Part model, mm, in its own coordinate system. Face numbers are marked on the shaded views. A direction names the side the tool comes from. Give positions to 0.01 mm unless a question says otherwise; leave off trailing zeros. Order: outer loops, then holes, each group sorted by start corner. A loop starts at its lowest first (then second) coordinate and runs counter-clockwise, first axis right, second up. Notation, with made-up numbers: (88, 82) -> (122, 82) arc R28 cw to (122, 107) -> close; hole circle Ø11 at (-32, 84). An arc over 180 degrees is marked (long way). Write item = value, one per line. Start each with the question number.
Item 1: Band-saw the part on D-D on y = -10. Write the cut outline in (x, z).
Item 2: Tool access for the marked faces 1 and 2: list every direction of +Z, -Z, +X, -X, +Y, -Y with a clear straight run to the whole face (end or side of a thin tool).
Item 3: Band-saw the part on C-C on z = 2. Count the separate pieces of the cut face and the enclosed holes in it, plus the area to 3 significant figures.
Item 4: Drill centre lines: line 1 along Y through (x, z) = (18.5, 1.5); line 2 along Y through (x, z) = (19.5, 1); line 3 along X through (y, z) = (6, 2.5). Where is each one in solid material? Low to high.
Item 5: Band-saw the part on A-A on y = 0. Write the cut outline in (x, z), plus the area to 3 significant figures.
Item 6: Flat gauge pins, fed straight in: P1, Ø5.5, axis at x = -19.05, y = 0, coming from the +Z side; P2, Ø3, axis at x = -21.5, z = 4, coming from the +Y side; P3, Ø2, axis at x = 13, y = 21.5, coming from the -Z side; P4, Ø7, axis at x = -3.5, y = -3, coming from the +Z side. Where does each tip first touch, or does it go through?
```python
from build123d import *

# Parameters (mm, degrees)
SKETCH1_R           = 30.5
SKETCH1_R_2         = 1.78
BOSS_EXTRUDE1_DEPTH = 3.1
SKETCH2_R           = 12.35
BOSS_EXTRUDE2_DEPTH = 4.1
SKETCH3_R           = 11.25
CUT_EXTRUDE1_DEPTH  = 1.5
SKETCH4_R           = 1.25
SKETCH4_R_2         = 3.1
CUT_EXTRUDE2_DEPTH  = 6.7


with BuildPart() as part:
    # Sketch1 → Boss-Extrude1 (new body)
    with BuildSketch(Plane.XY):
        Circle(SKETCH1_R)
        with Locations((0, 19.05)):
            Circle(SKETCH1_R_2, mode=Mode.SUBTRACT)
        with Locations((19.05, 0)):
            Circle(SKETCH1_R_2, mode=Mode.SUBTRACT)
        with Locations((0, -19.05)):
            Circle(SKETCH1_R_2, mode=Mode.SUBTRACT)
        with Locations((-19.05, 0)):
            Circle(SKETCH1_R_2, mode=Mode.SUBTRACT)
        with Locations((17.960512242, 17.960512242)):
            Circle(SKETCH1_R_2, mode=Mode.SUBTRACT)
        with Locations((17.960512242, -17.960512242)):
            Circle(SKETCH1_R_2, mode=Mode.SUBTRACT)
        with Locations((-17.960512242, -17.960512242)):
            Circle(SKETCH1_R_2, mode=Mode.SUBTRACT)
        with Locations((-17.960512242, 17.960512242)):
            Circle(SKETCH1_R_2, mode=Mode.SUBTRACT)
    extrude(amount=BOSS_EXTRUDE1_DEPTH)

    # Sketch2 → Boss-Extrude2 (add)
    with BuildSketch(Plane.XY.offset(3.1)):
        Circle(SKETCH2_R)
    extrude(amount=BOSS_EXTRUDE2_DEPTH)

    # Sketch3 → Cut-Extrude1 (cut)
    with BuildSketch(Plane.XY.offset(7.2)):
        Circle(SKETCH3_R)
    extrude(amount=-CUT_EXTRUDE1_DEPTH, mode=Mode.SUBTRACT)

    # Sketch4 → Cut-Extrude2 (cut, through all)
    with BuildSketch(Plane.XY.offset(5.7)):
        with Locations((5.656854249, 5.656854249)):
            Circle(SKETCH4_R)
        with Locations((5.656854249, -5.656854249)):
            Circle(SKETCH4_R)
        with Locations((-5.656854249, -5.656854249)):
            Circle(SKETCH4_R)
        with Locations((-5.656854249, 5.656854249)):
            Circle(SKETCH4_R)
        Circle(SKETCH4_R_2)
    extrude(amount=-CUT_EXTRUDE2_DEPTH, mode=Mode.SUBTRACT)


solid = part.part
```
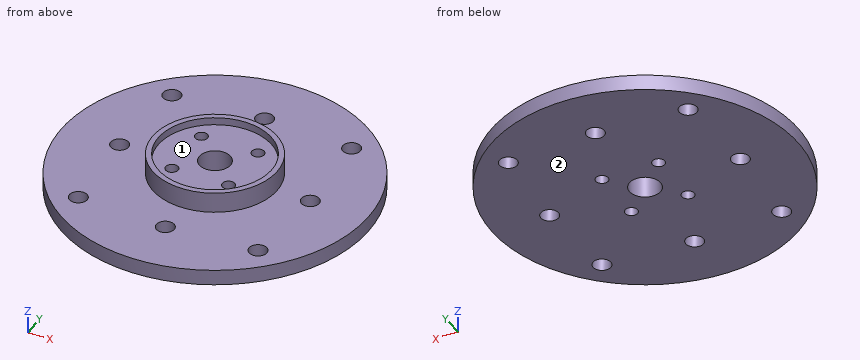
Values found:
q1.outline = (-28.81, 0) -> (28.81, 0) -> (28.81, 3.1) -> (7.25, 3.1) -> (7.25, 7.2) -> (5.15, 7.2) -> (5.15, 5.7) -> (-5.15, 5.7) -> (-5.15, 7.2) -> (-7.25, 7.2) -> (-7.25, 3.1) -> (-28.81, 3.1) -> close
q2.face_1 = +Z
q2.face_2 = -Z, +X, -X, +Y, -Y
q3.separate_pieces = 1
q3.enclosed_holes = 13
q3.area = 2,790 mm^2
q4.line_1 = -24.25 to -19.66, -16.26 to -1.69, 1.69 to 16.26, 19.66 to 24.25
q4.line_2 = -23.45 to -18.85, -17.07 to -1.72, 1.72 to 17.07, 18.85 to 23.45
q4.line_3 = -29.9 to -6.86, -4.45 to 4.45, 6.86 to 29.9
q5.outline = (-30.5, 0) -> (-20.83, 0) -> (-20.83, 3.1) -> (-30.5, 3.1) -> close; (-17.27, 0) -> (-3.1, 0) -> (-3.1, 5.7) -> (-11.25, 5.7) -> (-11.25, 7.2) -> (-12.35, 7.2) -> (-12.35, 3.1) -> (-17.27, 3.1) -> close; (3.1, 0) -> (17.27, 0) -> (17.27, 3.1) -> (12.35, 3.1) -> (12.35, 7.2) -> (11.25, 7.2) -> (11.25, 5.7) -> (3.1, 5.7) -> close; (20.83, 0) -> (30.5, 0) -> (30.5, 3.1) -> (20.83, 3.1) -> close
q5.area = 199 mm^2
q6.P1 = 3.1
q6.P2 = 22.76
q6.P3 = 0
q6.P4 = 5.7
